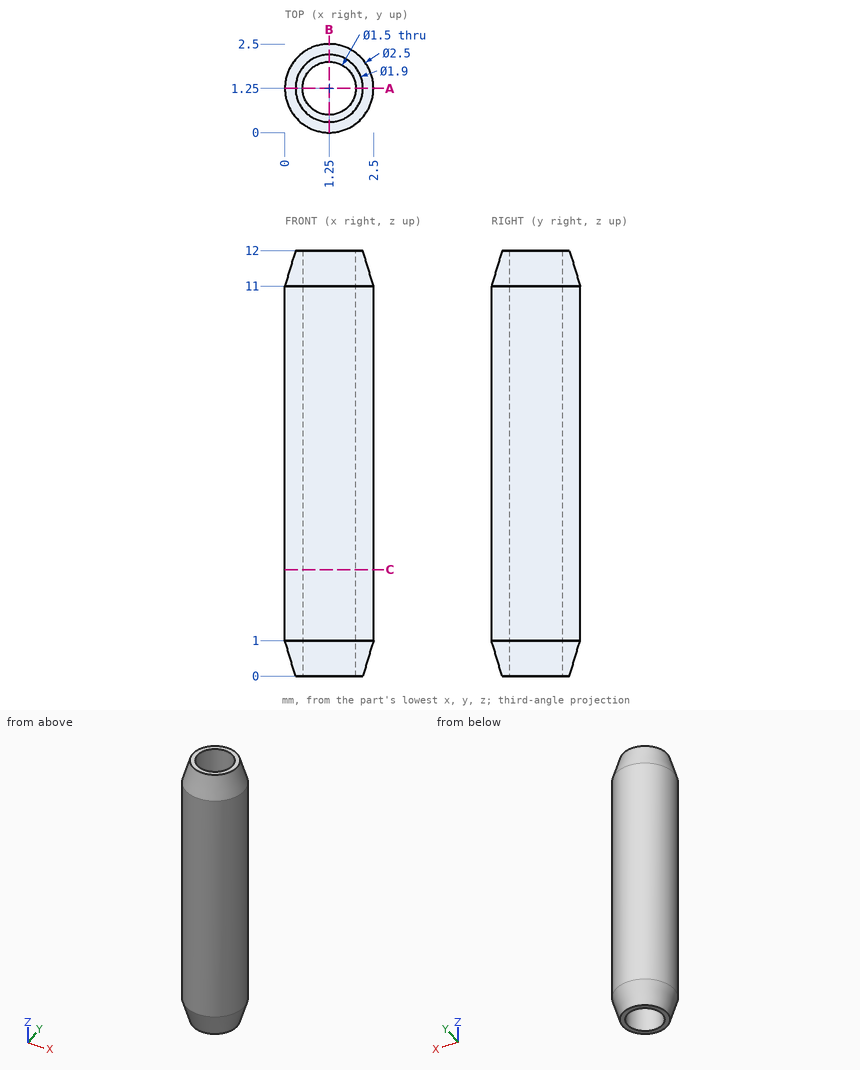
Here's the drawing with two shaded views (mm, measured from the low corner). I have some questions. Round coordinates to 2 decimals unless told otherwise and drop trailing zeros. Loops run counter-clockwise (first coordinate to the right, second up) from the corner with the lowest first, then second, coordinate; pieces in that order, holes last.
Item 1: Suppose I cut it at C-C, the plane z = 3. Write out the boundary of the cut face in (x, y), then the cut area to 3 significant figures.
Item 2: Please list where these lines run through material, in increasing order: L1, parallel to Y at x = 1.25, z = 9.25; L2, parallel to Y at x = 1.65, z = 1; L3, parallel to X at y = 0.95, z = 6.5.
Item 3: Suppose I cut it at A-A, the plane y = 1.25. Write out the boundary of the cut face in (x, z), then the cut area to 3 significant figures.
Item 4: Will this pin go through, and if not, where does the flat tip stop? pin 1 Ø1.2 at (x, y) = (1.25, 1.25) entering from -Z.
Reported:
1. outline: circle Ø2.5 at (1.25, 1.25); hole circle Ø1.5 at (1.25, 1.25)
1. area: 3.14 mm2
2. L1: y = 0 to 0.5, 2 to 2.5
2. L2: y = 0.07 to 0.62, 1.88 to 2.43
2. L3: x = 0.04 to 0.56, 1.94 to 2.46
3. outline: (0, 1) - (0.3, 0) - (0.5, 0) - (0.5, 12) - (0.3, 12) - (0, 11) - close; (2, 0) - (2.2, 0) - (2.5, 1) - (2.5, 11) - (2.2, 12) - (2, 12) - close
3. area: 11.4 mm2
4. pin 1: passes through
